```python
from build123d import *

# Parameters (mm, degrees)
EXTRUDE_1_DEPTH     = 30
SKETCH_2_R          = 4.25
CUT_EXTRUDE_1_DEPTH = 30
FILLET_1_R          = 10
FILLET_2_R          = 5
SKETCH_5_W          = 7
SKETCH_5_H          = 7
CUT_EXTRUDE_2_DEPTH = 20
FILLET_5_R          = 1
SKETCH_6_R          = 7
SKETCH_6_R_2        = 4.25
EXTRUDE_2_DEPTH     = 4


with BuildPart() as part:
    # 草图1 → 凸台-拉伸1 (new body)
    with BuildSketch(Plane.XY):
        Polygon((-4.331983806, 33.724696356), (-13.331983806, 6.619433198), (-13.331983806, -1.275303644), (-14.331983806, -1.275303644), (-14.331983806, -31.275303644), (5.668016194, -31.275303644), (5.668016194, 33.724696356), align=None)
    extrude(amount=EXTRUDE_1_DEPTH)

    # 草图2 → 切除-拉伸1 (cut)
    with BuildSketch(Plane.ZY.offset(14.331983806)):
        with Locations(Location((15, -16.275303644, 0), (0, 0, 270))):
            Circle(SKETCH_2_R)
    extrude(amount=-CUT_EXTRUDE_1_DEPTH, mode=Mode.SUBTRACT)

    # 圆角1
    fillet_1_edges = [part.edges().sort_by_distance(p)[0] for p in [
        (-13.331983806, 6.619433198, 15),
    ]]
    fillet(fillet_1_edges, radius=FILLET_1_R)

    # 圆角2
    fillet_2_edges = [part.edges().sort_by_distance(p)[0] for p in [
        (-4.331983806, 33.724696356, 15),
    ]]
    fillet(fillet_2_edges, radius=FILLET_2_R)

    # 草图5 → 切除-拉伸2 (cut)
    with BuildSketch(Plane.XY.offset(30)):
        with Locations((-10.831983806, -4.775303644)):
            Rectangle(SKETCH_5_W, SKETCH_5_H)
    extrude(amount=-CUT_EXTRUDE_2_DEPTH, mode=Mode.SUBTRACT)

    # 圆角5
    fillet_5_edges = [part.edges().sort_by_distance(p)[0] for p in [
        (-10.331983806, -1.275303644, 10),
        (-7.331983806, -4.775303644, 10),
        (-7.331983806, -1.275303644, 20),
        (-10.831983806, -8.275303644, 10),
        (-7.331983806, -8.275303644, 20),
    ]]
    fillet(fillet_5_edges, radius=FILLET_5_R)

    # 草图6 → 凸台-拉伸2 (add)
    with BuildSketch(Plane(origin=(5.668016194, 0, 0), x_dir=(0, 0, -1), z_dir=(1, 0, 0))):
        with Locations(Location((-15, -16.275303644, 0), (0, 0, 270))):
            Circle(SKETCH_6_R)
        with Locations(Location((-15, -16.275303644, 0), (0, 0, 270))):
            Circle(SKETCH_6_R_2, mode=Mode.SUBTRACT)
    extrude(amount=EXTRUDE_2_DEPTH)


solid = part.part
```
Input: part model. Units: mm. Frame: model coordinates. A direction names the side the tool comes from. Round coordinates to 2 decimals unless told otherwise and drop trailing zeros. Loops run counter-clockwise (first coordinate to the right, second up) from the corner with the lowest first, then second, coordinate; pieces in that order, holes last.
1) Section query D-D on x = 7. Return the cut outline in (y, z).
Ans:
outline: circle Ø14 at (-16.28, 15); hole circle Ø8.5 at (-16.28, 15)
2) Section query B-B on x = 2. Return the cut outline in (y, z), plus the area to 3 significant figures.
Ans:
outline: (-31.28, 0) - (33.72, 0) - (33.72, 30) - (-31.28, 30) - close; hole circle Ø8.5 at (-16.28, 15)
area: 1,890 mm2
3) Set-up query: faces 1 (the flat face through (-4, -31.275, 15)), 2 (the cylindrical face through (7.64, -14.758, 21.834)), 3 (the flat face through (-11, -8.275, 21)). Return all of +Z, -Z, +X, -X, +Y, -Y with unobstructed straight access to the full face (end or side cutting, diameter ignored); none if empty.
Ans:
face 1: +Z, -Z, +X, -X, -Y
face 2: +X
face 3: +Z, -X
4) Section query A-A on z = 15. Return the cut outline in (x, y).
Ans:
outline: (-14.33, -31.28) - (5.67, -31.28) - (5.67, -23.28) - (9.67, -23.28) - (9.67, -20.53) - (-14.33, -20.53) - close; (-14.33, -12.03) - (9.67, -12.03) - (9.67, -9.28) - (5.67, -9.28) - (5.67, 33.72) - (-0.72, 33.72) arc R5 ccw to (-5.47, 30.3) - (-12.82, 8.15) arc R10 ccw to (-13.33, 5) - (-13.33, -1.28) - (-8.33, -1.28) arc R1 cw to (-7.33, -2.28) - (-7.33, -7.28) arc R1 cw to (-8.33, -8.28) - (-14.33, -8.28) - close
5) Pull-direction query (Y, two-part tool) for faces 4 (the flat face through (-7.332, -5, 21)), 5 (the flat face through (-9.094, 19.382, 14.79)), 6 (the flat face through (-13.332, 1, 15)); classes: released by +Y, released by -Y, zero draft, split by the parting line, or undercut.
Ans:
face 4: undercut
face 5: released by +Y
face 6: zero draft
6) Section query C-C on z = 25.5. Return the cut outline in (x, y), plus the area to 3 significant figures.
Ans:
outline: (-14.33, -31.28) - (5.67, -31.28) - (5.67, 33.72) - (-0.72, 33.72) arc R5 ccw to (-5.47, 30.3) - (-12.82, 8.15) arc R10 ccw to (-13.33, 5) - (-13.33, -1.28) - (-8.33, -1.28) arc R1 cw to (-7.33, -2.28) - (-7.33, -7.28) arc R1 cw to (-8.33, -8.28) - (-14.33, -8.28) - close
area: 1,090 mm2
7) Pin query (flat end, axial travel): pin 1 (2 mm diameter, centred on x = 7, y = 3, fed in from +Z); pin 2 (3 mm diameter, centred on y = 4.5, z = 13, fed in from -X); pin 3 (3 mm diameter, centred on x = -11.5, y = -5.5, fed in from +Z); pin 4 (0.8 mm diameter, centred on x = -14, z = 2.5, fed in from +Y). Return the tip coordinate at first contact, or that it passes through.
Ans:
pin 1: passes through
pin 2: stops at x = -13.33
pin 3: stops at z = 10
pin 4: stops at y = -1.28
8) Material intervals for line 1 (X direction, y = -4, z = 28.75); line 2 (X direction, y = -27, z = 24.75); line 3 (Y direction, x = 1.25, z = 15), sorted ascending.
Ans:
line 1: x = -7.33 to 5.67
line 2: x = -14.33 to 5.67
line 3: y = -31.28 to -20.53, -12.03 to 33.72
